```python
from build123d import *

# Parameters (mm, degrees)
F0_R         = 2.125
F1_DEPTH     = 5
F3_DEPTH     = 20
F5_DEPTH     = 15
F6_SIZE      = 10
F7_R         = 2.125
F8_DEPTH     = 5
F9_R         = 2.125
F10_DEPTH    = 5
F11_W        = 40
F11_H        = 20
F11_R        = 2.125
F12_DEPTH    = 24
F14_DEPTH    = 25
F15_R        = 4.25
F16_DEPTH    = 20
F17_R        = 3.5
F18_DEPTH    = 25
F19_W        = 20
F19_H        = 24
F20_DEPTH    = 5
F22_DEPTH    = 12.5
F23_T4_DEPTH = 20
F23_S5_R     = 2.125
F23_T6_DEPTH = 12
F23_T7_DEPTH = 38.2168298797
F23_T9_DEPTH = 20.3584149398
F24_R        = 3.5
F25_DEPTH    = 44.001
F26_R        = 4.25
F26_R_2      = 1.6
F27_DEPTH    = 5
F28_R        = 2.125
F29_DEPTH    = 40.001
F31_DEPTH    = 4
F32_R        = 3.5
F33_DEPTH    = 4


# Not quite as in the source:
# - a fillet or chamfer that OpenCascade refuses, or shapes differently, is made with other operations: its cross-section is extruded or revolved along the edge and cut away or added


with BuildPart() as f1:
    # F0 (on Top) → F1 (new body)
    with BuildSketch(Plane.XY):
        Polygon((0, 20), (0, 40), (-20, 40), (-20, 0), (20, 0), (20, 20), align=None)
        with Locations((-7.5, 12.5)):
            Circle(F0_R, mode=Mode.SUBTRACT)
        with Locations((10, 12.5)):
            Circle(F0_R, mode=Mode.SUBTRACT)
        with Locations((-7.5, 30)):
            Circle(F0_R, mode=Mode.SUBTRACT)
    extrude(amount=F1_DEPTH)

    # F2 (on face) → F3 (join)
    with BuildSketch(Plane.XY.offset(5)):
        Polygon((-15, 40), (-20, 40), (-20, 0), (20, 0), (20, 5), (-15, 5), align=None)
    extrude(amount=F3_DEPTH)

    # F4 (on face) → F5 (join)
    with BuildSketch(Plane.XY.offset(25)):
        Polygon((-15, 5), (-15, 25), (-20, 25), (-20, 0), (5, 0), (5, 5), align=None)
    extrude(amount=F5_DEPTH)

    # F6
    f6_edges = [f1.edges().sort_by_distance(p)[0] for p in [
        (0, 20, 2.5),
        (-17.5, 25, 25),
        (5, 2.5, 25),
    ]]
    chamfer(f6_edges, length=F6_SIZE)

    # F7 (on face) → F8 (cut)
    with BuildSketch(Plane.XZ):
        with Locations((-7.5, 32.5)):
            Circle(F7_R)
        with Locations((10, 12.5)):
            Circle(F7_R)
    extrude(amount=-F8_DEPTH, mode=Mode.SUBTRACT)

    # F9 (on face) → F10 (cut)
    with BuildSketch(Plane(origin=(-20, 0, 0), x_dir=(0, -1, 0), z_dir=(-1, 0, 0))):
        with Locations((-12.5, 32.5)):
            Circle(F9_R)
        with Locations((-30, 12.5)):
            Circle(F9_R)
    extrude(amount=-F10_DEPTH, mode=Mode.SUBTRACT)

    # F11 (on face) → F12 (join)
    with BuildSketch(Plane(origin=(0, 0, 0), x_dir=(1, 0, 0), z_dir=(0, 0, -1))):
        with Locations((0, -10)):
            Rectangle(F11_W, F11_H)
        with Locations((-7.5, -12.5)):
            Circle(F11_R, mode=Mode.SUBTRACT)
        with Locations((10, -12.5)):
            Circle(F11_R, mode=Mode.SUBTRACT)
    extrude(amount=F12_DEPTH)

    # F13 (on face) → F14 (cut)
    with BuildSketch(Plane(origin=(0, 20, 0), x_dir=(-1, 0, 0), z_dir=(0, 1, 0))):
        Polygon((0, -24), (0, -11.5), (0, 0), (-20, 0), (-20, -24), align=None)
    extrude(amount=-F14_DEPTH, mode=Mode.SUBTRACT)

    # F15 (on face) → F16 (cut)
    with BuildSketch(Plane.YZ):
        with Locations((12.5, -12.5)):
            Circle(F15_R)
    extrude(amount=-F16_DEPTH, mode=Mode.SUBTRACT)

    # F17 (on face) → F18 (cut)
    with BuildSketch(Plane(origin=(0, 0, -24), x_dir=(1, 0, 0), z_dir=(0, 0, -1))):
        with Locations((-7.5, -12.5)):
            Circle(F17_R)
    extrude(amount=-F18_DEPTH, mode=Mode.SUBTRACT)

    # F19 (on face) → F20 (join)
    with BuildSketch(Plane(origin=(0, 20, 0), x_dir=(-1, 0, 0), z_dir=(0, 1, 0))):
        with Locations((10, -12)):
            Rectangle(F19_W, F19_H)
    extrude(amount=F20_DEPTH)

    # F21 (on face) → F22 (join)
    with BuildSketch(Plane(origin=(-20, 0, 0), x_dir=(0, -1, 0), z_dir=(-1, 0, 0))):
        Polygon((-17.25, -24), (-25, -24), (-25, -44), (0, -44), (0, -24), (-7.75, -24), (-7.75, -39), (-17.25, -39), align=None)
    extrude(amount=-F22_DEPTH)

    # F23: chamfer of 5 on 5 edges, made by hand


with BuildPart() as f23_tool2:
    # F23_s3 → F23_t4 (new body)
    with BuildSketch(Plane.YZ.offset(-20)):
        Polygon((25, -5), (30, 0), (25, 0), align=None)
    extrude(amount=F23_T4_DEPTH)

    # F23_s5 → F23_t6 (cut, symmetric)
    with BuildSketch(Plane.XY.offset(-2.5)):
        with Locations((-7.5, 30)):
            Circle(F23_S5_R)
    extrude(amount=F23_T6_DEPTH, both=True, mode=Mode.SUBTRACT)


with BuildPart() as f1_1:
    add(f1.part)

    # F23_t1: union F23_tool2
    add(f23_tool2.part)

    # F23_s8 → F23_t7 (cut)
    with BuildSketch(Plane.YZ.offset(-32.8584149398)):
        Polygon((25, -39), (20, -44), (25, -44), align=None)
        Polygon((0, -39), (5, -44), (0, -44), align=None)
    extrude(amount=F23_T7_DEPTH, mode=Mode.SUBTRACT)

    # F23_s10 → F23_t9 (cut)
    with BuildSketch(Plane.YZ.offset(-7.5)):
        Polygon((5, -24), (0, -19), (0, -24), align=None)
        Polygon((25, -19), (20, -24), (25, -24), align=None)
    extrude(amount=F23_T9_DEPTH, mode=Mode.SUBTRACT)

    # F24 (on face) → F25 (cut, through all)
    with BuildSketch(Plane(origin=(0, 0, 0), x_dir=(1, 0, 0), z_dir=(0, 0, -1))):
        with Locations((-7.5, -30)):
            Circle(F24_R)
    extrude(amount=F25_DEPTH, mode=Mode.SUBTRACT)

    # F26 (on face) → F27 (join)
    with BuildSketch(Plane(origin=(-20, 0, 0), x_dir=(0, -1, 0), z_dir=(-1, 0, 0))):
        with Locations((-12.5, -12.5)):
            Circle(F26_R)
        with Locations((-12.5, -12.5)):
            Circle(F26_R_2, mode=Mode.SUBTRACT)
    extrude(amount=-F27_DEPTH)

    # F28 (on face) → F29 (cut, through all)
    with BuildSketch(Plane.XZ):
        with Locations((-13.75, -31.5)):
            Circle(F28_R)
    extrude(amount=-F29_DEPTH, mode=Mode.SUBTRACT)

    # F30 (on face) → F31 (cut)
    with BuildSketch(Plane.XZ):
        Polygon((-10.825, -33.1887495374), (-10.825, -29.8112504626), (-13.75, -28.1225009252), (-16.675, -29.8112504626), (-16.675, -33.1887495374), (-13.75, -34.8774990748), align=None)
    extrude(amount=-F31_DEPTH, mode=Mode.SUBTRACT)

    # F32 (on face) → F33 (cut)
    with BuildSketch(Plane(origin=(0, 25, 0), x_dir=(-1, 0, 0), z_dir=(0, 1, 0))):
        with Locations((13.75, -31.5)):
            Circle(F32_R)
    extrude(amount=-F33_DEPTH, mode=Mode.SUBTRACT)


solid = f1_1.part
```
Model file for the job. Use its own axes, mm. A direction names the side the tool comes from. Coordinates: 2 decimals unless noted, no trailing zeros. Loops run counter-clockwise (first coordinate to the right, second up) from the corner with the lowest first, then second, coordinate; pieces in that order, holes last. Notation, with made-up numbers: (12.25, 77.25) - (32.25, 77.25) arc R12 ccw to (32.25, 95.25) - close; hole circle Ø1 at (42, 24.25). An arc over 180 degrees is marked (long way). Answer as a JSON object with one key per item and string values. Group by question number.
(1) Cut at C-C (z = -12.5). Give the cut face in (x, y).
(2) Cut at A-A (z = -31.5). Give the cut face in (x, y) (3 decimals), then the cut area to 3 significant figures.
(3) Cut at B-B (z = 32.5). Give the cut face in (x, y) (3 decimals), then the cut area to 4 significant figures.
(4) Tool access for faces 5 (the face through (-12, 12, -24)), 6 (the face through (-4, 23, -21)), 7 (the face through (-15, 18, 22)), 8 (the face through (5, 2, 37)), 9 (the face through (-10.825, 2, -32)): list every direction of +Z, -Z, +X, -X, +Y, -Y with a clear straight run to the whole face (end or side of a thin tool).
(5) Flat gauge pins, fed straight in: pin 1 (7 mm diameter, centred on x = -7.5, y = 30, fed in from +Z); pin 2 (3 mm diameter, centred on y = 12.5, z = -12.5, fed in from -X) (3 decimals); pin 3 (10 mm diameter, centred on x = 7, y = 21.5, fed in from -Z); pin 4 (7 mm diameter, centred on y = 12.5, z = 32.5, fed in from +X). Where does each tip first touch, or does it go through?
(6) Two-plate mould, pull along Y, no slides. Class faces 1 (the face through (-14, 12, -39)), 2 (the face through (-15.233, 1.972, -34.021)), 3 (the face through (-6.519, 28.115, 2.535)), 4 (the face through (-17, 30, 30)): released by +Y, released by -Y, zero draft, split by the parting line, or undercut.
(7) Probe line 1 along Z through (x, y) = (-16.9, 30) (3 decimals); line 2 along X through (y, z) = (12.5, -2.5); line 3 along Y through (x, z) = (16, 15.5). List the from-to ranges inside material, lowest first.
(8) Cut at D-D (y = 23). Give the cut face in (x, z), then the cut area to 3 significant figures.
Geometry says:
{
 "1": {"outline": "(-20, 0) - (0, 0) - (0, 8.25) - (-15, 8.25) - (-15, 10.9) - (-20, 10.9) - close; (-20, 14.1) - (-15, 14.1) - (-15, 16.75) - (0, 16.75) - (0, 25) - (-20, 25) - close"},
 "2": {"outline": "(-20, 0) - (-16.675, 0) - (-16.675, 4) - (-15.875, 4) - (-15.875, 7.75) - (-20, 7.75) - close; (-20, 17.25) - (-15.875, 17.25) - (-15.875, 21) - (-17.25, 21) - (-17.25, 25) - (-20, 25) - close; (-11.625, 4) - (-10.825, 4) - (-10.825, 0) - (-7.5, 0) - (-7.5, 7.75) - (-11.625, 7.75) - close; (-11.625, 17.25) - (-7.5, 17.25) - (-7.5, 25) - (-10.25, 25) - (-10.25, 21) - (-11.625, 21) - close", "area": "110 mm^2"},
 "3": {"outline": "(-20, 0) - (-9.625, 0) - (-9.625, 5) - (-15, 5) - (-15, 10.375) - (-20, 10.375) - close; (-20, 14.625) - (-15, 14.625) - (-15, 27.5) - (-20, 27.5) - close; (-5.375, 0) - (7.5, 0) - (7.5, 5) - (-5.375, 5) - close", "area": "207.5 mm^2"},
 "4": {"face 5": "+X", "face 6": "-Z, +X, +Y", "face 7": "+Z, +X, +Y", "face 8": "+Z, +X, +Y, -Y", "face 9": "-Y"},
 "5": {"pin 1": "stops at z = 5", "pin 2": "passes through", "pin 3": "stops at z = 0", "pin 4": "stops at x = -15"},
 "6": {"face 1": "undercut", "face 2": "zero draft", "face 3": "undercut", "face 4": "released by +Y"},
 "7": {"line 1": "z = 0 to 10.375, 14.625 to 30", "line 2": "x = -20 to -11, -4 to 0", "line 3": "y = 0 to 5"},
 "8": {"outline": "(-20, -41) - (-7.5, -41) - (-7.5, -21) - (0, -21) - (0, 0) - (7, 0) - (7, 5) - (-15, 5) - (-15, 40) - (-20, 40) - close; hole circle Ø7 at (-13.75, -31.5)", "area": "942 mm^2"}
}
